Source: three-view drawing plus pictorial views. Frame: mm from the lowest corner of the part. A direction names the side the tool comes from. Coordinates: 2 decimals unless noted, no trailing zeros. Order: outer loops, then holes, each group sorted by start corner. A loop starts at its lowest first (then second) coordinate and runs counter-clockwise, first axis right, second up. Notation, with made-up numbers: M 67.25,28 L 89.25,28 A25 ccw 89.25,54 Z; hole C -28,-29.5 d8. An arc over 180 degrees is marked long. One line per question, with ' | ' between items.
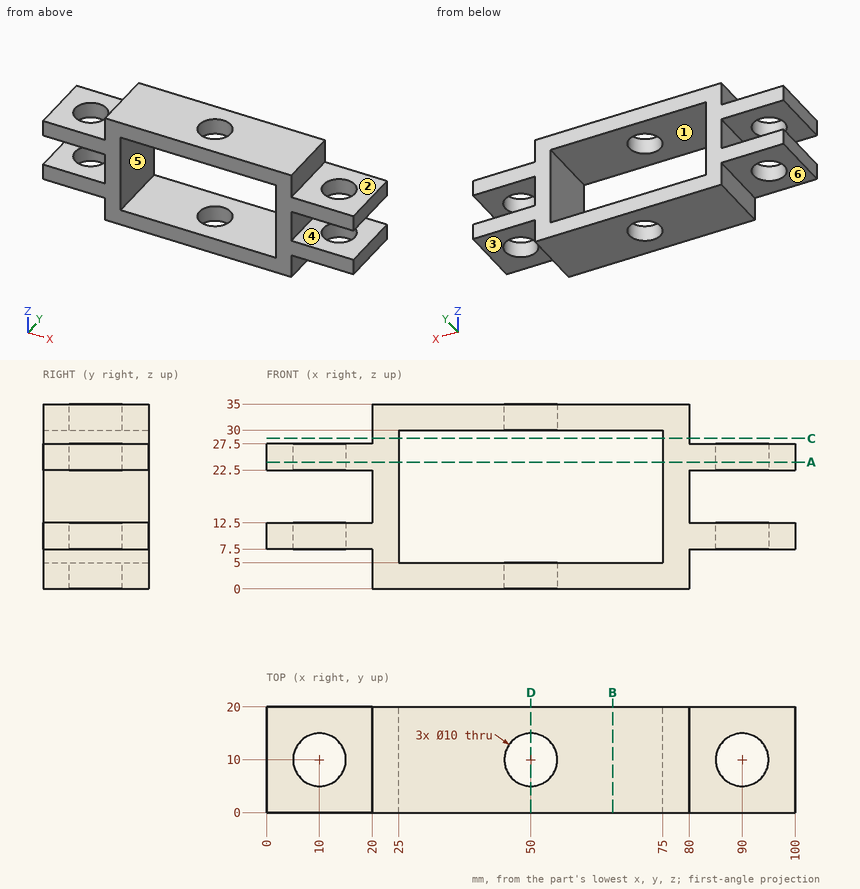
1. Section D-D, the plane x = 50. Output: boundary loops of the cut face in (y, z), and give its area (3 significant figures).
Response values:
outline: M 0,0 L 5,0 L 5,5 L 0,5 Z; M 0,30 L 5,30 L 5,35 L 0,35 Z; M 15,0 L 20,0 L 20,5 L 15,5 Z; M 15,30 L 20,30 L 20,35 L 15,35 Z | area: 100 mm^2
2. Material intervals for line 1 (Z direction, x = 68, y = 13); line 2 (Y direction, x = 50, z = 33.35); line 3 (X direction, y = 4, z = 12), sorted ascending. Write a range as [from, to].
Response values:
line 1: z = [0, 5], [30, 35] | line 2: y = [0, 5], [15, 20] | line 3: x = [0, 25], [75, 100]
3. Pin query (flat end, axial travel): P1, Ø2, axis at y = 6, z = 4, coming from the -X side; P2, Ø3, axis at x = 14.5, y = 11, coming from the -Z side; P3, Ø4, axis at y = 14, z = 32.5, coming from the +X side; P4, Ø6, axis at x = 90, y = 10, coming from the +Z side. Return the tip coordinate at first contact, or that it passes through.
Response values:
P1: stops at x = 20 | P2: stops at z = 7.5 | P3: stops at x = 80 | P4: passes through
4. Section B-B, the plane x = 65.5. Output: boundary loops of the cut face in (y, z), and give its area (3 significant figures).
Response values:
outline: M 0,0 L 20,0 L 20,5 L 0,5 Z; M 0,30 L 20,30 L 20,35 L 0,35 Z | area: 200 mm^2
5. Draft query along Z for the marked faces 1, 2 and 3. Return one class per face: pulls with the +Z half, pulls with the -Z half, needs draft (parallel to the pull), parting line crosses it, or undercut.
Response values:
face 1: undercut | face 2: pulls with the +Z half | face 3: pulls with the -Z half
6. Access query for the marked faces 4, 5 and 6. Directions: +Z, -Z, +X, -X, +Y, -Y. A direction counts if a zero-diameter tool reaches every point of the face in a straight line with its end or side. Return the directions, or none.
Response values:
face 4: +X, +Y, -Y | face 5: +Y, -Y | face 6: -Z, -X, +Y, -Y
7. Section A-A, the plane z = 24. Output: boundary loops of the cut face in (x, y).
Response values:
outline: M 0,0 L 25,0 L 25,20 L 0,20 Z; M 75,0 L 100,0 L 100,20 L 75,20 Z; hole C 10,10 d10; hole C 90,10 d10
8. Section C-C, the plane z = 28.5. Output: boundary loops of the cut face in (x, y), and give its area (3 significant figures).
Response values:
outline: M 20,0 L 25,0 L 25,20 L 20,20 Z; M 75,0 L 80,0 L 80,20 L 75,20 Z | area: 200 mm^2
